Autodesk Inventor part; units mm, degrees
ref_plane "Work Plane1" through (-16.4338, 3.9733, 0) normal (0, 1, 0) x (1, 0, 0)
ref_plane "Work Plane2" through (-16.4338, -4.9929, 0) normal (0, -1, 0) x (1, 0, 0)
ref_plane "Work Plane3" through (-16.4338, -3.0722, 0) normal (0, 1, 0) x (1, 0, 0)
sketch "Sketch1" plane through (0, 0, 0) normal (0, 0, 1) x (1, 0, 0)
  line L0 (-27.5463, 4.2273) -> (-26.0223, 4.2273)
  line L1 (-26.0223, 4.2273) -> (-26.0223, -5.2469)
  line L2 (-26.0223, -5.2469) -> (-27.5463, -5.2469)
  line L3 (-27.5463, -5.2469) -> (-27.5463, 4.2273)
  line L4 (-16.4338, 9.0278) -> (-16.4338, -15.3549)
  dimension "d0" = 9.4742
  dimension "d1" = 1.524
  dimension "d2" = 11.1125
revolve "Revolution1" add sketch "Sketch1" angle 360 about axis through (-16.4338, 9.0278, 0) along (0, -1, 0)
ref_plane "Work Plane1" through (-16.4338, 3.9733, 0) normal (0, 1, 0) x (1, 0, 0)
sketch "Sketch2" plane through (-16.4338, 3.9733, 0) normal (0, 1, 0) x (1, 0, 0)
  circle A0 centre (0, 0) radius 11.1125
  circle A1 centre (0, 0) radius 6.35
  dimension "d5" = 12.7
  dimension "d35" = 22.225
extrude "Extrusion1" add sketch "Sketch2" against normal blind 1.9207
ref_plane "Work Plane2" through (-16.4338, -4.9929, 0) normal (0, -1, 0) x (1, 0, 0)
sketch "Sketch3" plane through (-16.4338, -4.9929, 0) normal (0, -1, 0) x (1, 0, 0)
  circle A0 centre (0, 0) radius 11.1125
  circle A1 centre (0, 0) radius 6.35
  dimension "d9" = 12.7
  dimension "d34" = 22.225
extrude "Extrusion2" add sketch "Sketch3" against normal blind 1.9207
ref_plane "Work Plane3" through (-16.4338, -3.0722, 0) normal (0, 1, 0) x (1, 0, 0)
sketch "Sketch4" plane through (-16.4338, -3.0722, 0) normal (0, 1, 0) x (1, 0, 0)
  circle A0 centre (0, 0) radius 10.3505
  dimension "d13" = 20.701
extrude "Extrusion3" cut sketch "Sketch4" along normal blind 5.1248
sketch "Sketch5" plane through (-16.4338, -4.9929, 0) normal (0, -1, 0) x (1, 0, 0)
  circle A0 centre (0, 0) radius 9.5885
  circle A1 centre (0, 0) radius 9.3345
  dimension "d16" = 0.254
extrude "Extrusion4" cut sketch "Sketch5" against normal blind 0.254
chamfer "Chamfer1" distance 0.254 angle 45 1 edges at (-25.7683, -4.9929, 0)
sketch "Sketch6" plane through (-16.4338, 3.9733, 0) normal (0, 1, 0) x (1, 0, 0)
  circle A0 centre (0, 0) radius 9.5885
  circle A1 centre (0, 0) radius 9.3345
  dimension "d22" = 0.254
extrude "Extrusion5" cut sketch "Sketch6" against normal blind 0.254
chamfer "Chamfer2" distance 0.254 angle 45 1 edges at (-25.7683, 3.9733, 0)
chamfer "Chamfer3" distance 0.254 angle 45 1 edges at (-5.3213, -5.2469, 0)
chamfer "Chamfer4" distance 0.254 angle 45 1 edges at (-5.3213, 4.2273, 0)
properties part number "Outer Casing 1764"
Verification items for the finished model (mm, model axes). A direction names the side the tool comes from. Round coordinates to 2 decimals unless told otherwise and drop trailing zeros. Order: outer loops, then holes, each group sorted by start corner. A loop starts at its lowest first (then second) coordinate and runs counter-clockwise, first axis right, second up.
1) Draft check along X on faces 5 (the flat face through (-12, -3.072, 5)), 6 (the cylindrical face through (-27.033, -0.447, 3.338)), 7 (the flat face through (-16, -5.247, 10)). Enter one of: +X half, -X half, draft (parallel to the pull), parting line (faces both ways), or undercut.
Geometry says:
face 5: undercut
face 6: parting line
face 7: draft
2) Tool access check on faces 1 (the cylindrical face through (-17.066, -4.996, -9.568)), 2 (the flat face through (-12, 2.053, -5)), 3 (the cylindrical face through (-21.473, -4.046, -3.864)), 4 (the flat face through (-23, 3.973, 2)). Record the directions out of +Z, -Z, +X, -X, +Y, -Y that give a thin tool (end or side, any length) a straight path to the whole face; none if there is none.
Geometry says:
face 1: -Y
face 2: none
face 3: +Y, -Y
face 4: +Y
3) Material ranges on line 1 (Y direction, x = -22.25, z = -4.5); line 2 (X direction, y = 2.95, z = 0); line 3 (X direction, y = 3.5, z = -0.75), recorded low to high.
Geometry says:
line 1: y = -4.99 to -3.07, 2.05 to 3.97
line 2: x = -27.55 to -22.78, -10.08 to -5.32
line 3: x = -27.52 to -22.74, -10.13 to -5.35
4) Depth check by flat-ended pin: pin 1 (10 mm diameter, centred on x = -16.43, z = 0, fed in from +Y); pin 2 (10.5 mm diameter, centred on x = -16.5, z = -3, fed in from -Y); pin 3 (9 mm diameter, centred on x = -19, z = 4, fed in from +Y); pin 4 (5 mm diameter, centred on y = 1, z = 5, fed in from +X). Enter the tip coordinate at first touch or a pass-through.
Geometry says:
pin 1: passes through
pin 2: stops at y = -4.99
pin 3: stops at y = 3.97
pin 4: stops at x = -5.61
5) Cross-section at A-A, the plane y = -2.5. Record the cut outline in (x, z) (1 decimal).
Geometry says:
outline: circle Ø22.2 at (-16.4, 0); hole circle Ø20.7 at (-16.4, 0)
